Can you work these out from the drawing? Everything is in mm from the part's minimum corner. A direction names the side the tool comes from. Give positions to 0.01 mm unless a question says otherwise; leave off trailing zeros. Loops run counter-clockwise (first coordinate to the right, second up) from the corner with the lowest first, then second, coordinate; pieces in that order, holes last. Notation, with made-up numbers: (-26, -23) -> (8, -23) arc R23 ccw to (8, -3) -> close; hole circle Ø8 at (-14.75, 62). An arc over 180 degrees is marked (long way). Return JSON: item names as keys, results as strings. Group by question number.
Q1. Which directions (+Z, -Z, +X, -X, +Y, -Y) give clear straight access to the entire face, cutting with the end or side of a thin tool? Please do the marked faces 1 and 2.
Q2. I need wall thicknesses on line 1 along Y through (x, z) = (8.25, 14.5) (1 decimal); line 2 along Z through (x, y) = (12.25, 13.25) (1 decimal); line 3 along Z through (x, y) = (12.5, 13) (1 decimal). Which ranges of each line are inside material? Lowest first, please. Write a range as [from, to].
Q3. Suppose I cut it at B-B, the plane z = 17. Please give me the cut outline in (x, y) (1 decimal), and give its area (3 significant figures).
Q4. Will these pins go through, and if not, where does the flat tip stop? pin 1 (8 mm diameter, centred on x = 9, y = 9.5, fed in from -Z); pin 2 (3 mm diameter, centred on x = 8.5, z = 55.5, fed in from -Y); pin 3 (3 mm diameter, centred on y = 13, z = 25.5, fed in from -X); pin 4 (5 mm diameter, centred on y = 11.5, z = 39, fed in from -X).
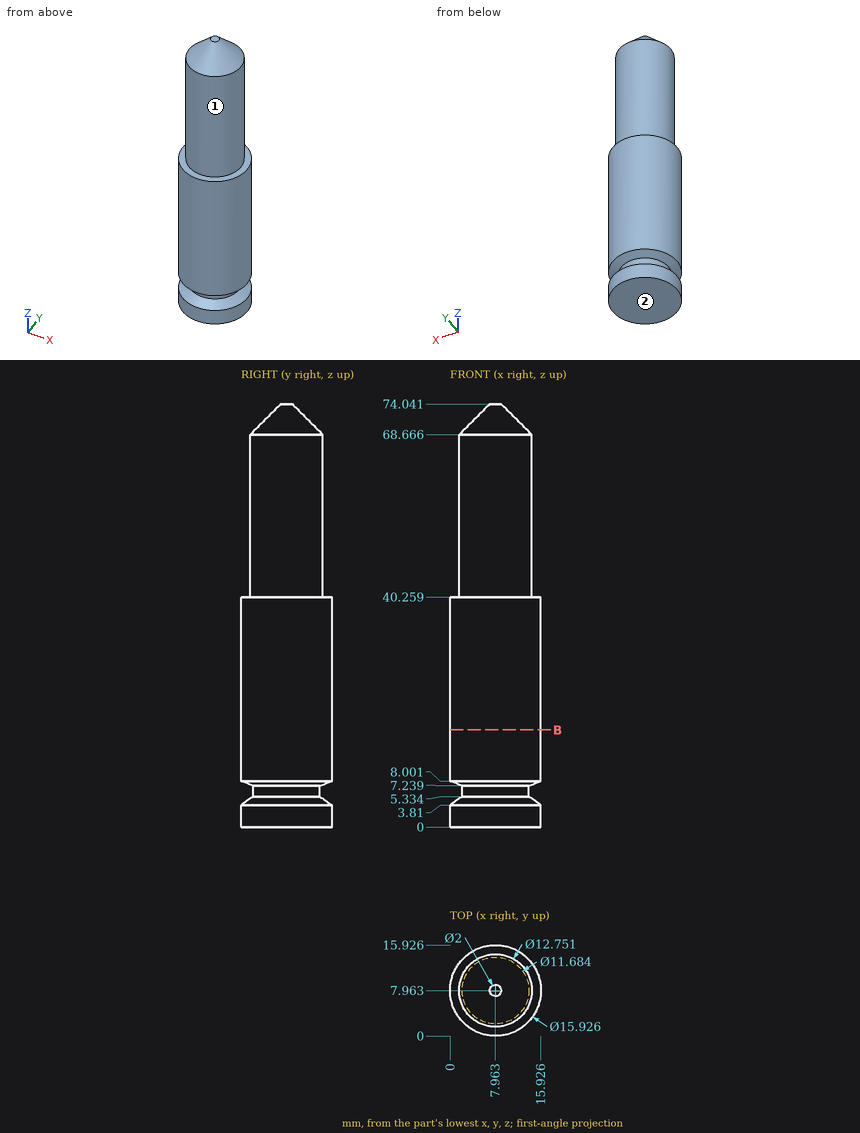
Ans:
{
 "1": {"face 1": "+Z", "face 2": "-Z, +X, -X, +Y, -Y"},
 "2": {"line 1": "y = [0, 15.9]", "line 2": "z = [0, 4.6], [7.6, 40.3]", "line 3": "z = [0, 4.7], [7.6, 40.3]"},
 "3": {"outline": "circle Ø15.9 at (8, 8)", "area": "199 mm^2"},
 "4": {"pin 1": "stops at z = 0", "pin 2": "stops at y = 1.59", "pin 3": "stops at x = 0.83", "pin 4": "stops at x = 0.07"}
}
